The model under review builds one solid part; all positions refer to its coordinate system, in mm. Face numbers are marked on the shaded views. A direction names the side the tool comes from. Round coordinates to 2 decimals unless told otherwise and drop trailing zeros. Order: outer loops, then holes, each group sorted by start corner. A loop starts at its lowest first (then second) coordinate and runs counter-clockwise, first axis right, second up.
1) Clearance check with flat-ended pins moving along their axes: P1, Ø1.5, axis at x = 8.5, z = -4.5, coming from the -Y side; P2, Ø4.5, axis at x = -2.5, y = 0, coming from the -Z side; P3, Ø3, axis at x = -5, z = 0, coming from the -Y side; P4, Ø4, axis at x = 19.5, y = 6, coming from the +Z side. State where each tip first meets the part, or that it passes through.
2) Consider section C-C (x = 25.5). Give the boundary of the cut face in (y, z), then the cut area to 3 significant figures.
3) Consider section D-D (y = 5.75). Give the boundary of the cut face in (x, z).
4) Machinability: for the marked faces 1, 2 and 3, which of the approach directions +Z, -Z, +X, -X, +Y, -Y give a long, thin tool a straight path to every point of the face, cutting with its end or side? Answer none if there is none.
5) To check wall thickness, follow L1, parallel to Z at x = -5, y = 0.75; L2, parallel to X at y = -2, z = 5.25; L3, parallel to Z at x = 17.5, y = -0.5. State the ranges of each line that lie inside material, in increasing order.
6) Mouldability with a two-part tool opening along X and no side actions: class the marked faces 4, 5 and 6 as pulls with the +X half, pulls with the -X half, needs draft (parallel to the pull), parting line crosses it, or undercut.
7) Consider section A-A (z = 0). Give the boundary of the cut face in (x, y).
8) Consider section B-B (y = 0). Give the boundary of the cut face in (x, z), then the cut area to 3 significant figures.
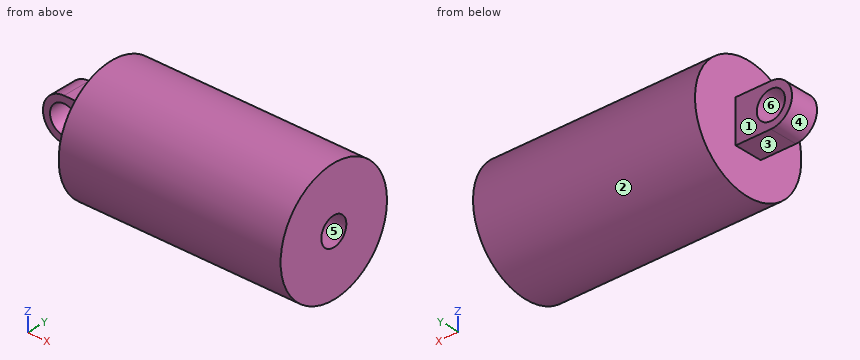
Autodesk Inventor part; units mm, degrees
ref_plane "YZ Plane" through (0, 0, 0) normal (1, 0, 0) x (0, 1, 0)
ref_plane "XZ Plane" through (0, 0, 0) normal (0, 1, 0) x (-1, 0, 0)
ref_plane "XY Plane" through (0, 0, 0) normal (0, 0, 1) x (1, 0, 0)
sketch "スケッチ1" plane through (0, 0, 0) normal (1, 0, 0) x (0, 1, 0)
  circle A0 centre (0, 0) radius 8.5
  dimension "d0" = 17
extrude "押し出し1" add sketch "スケッチ1" along normal blind 31.5
sketch "スケッチ2" plane through (0, 0, 0) normal (0, 1, 0) x (-1, 0, 0)
  circle A0 centre (5, 0) radius 2
  circle A1 centre (5, 0) radius 3
  line L0 (0, 0) -> (0, 5.5308)
  line L1 (0, 5.5308) -> (0, -7.9673)
  line L2 (5, 3) -> (0, 3)
  line L3 (5, -3) -> (0, -3)
  dimension "d3" = 4
  dimension "d4" = 5
  dimension "d5" = 6
extrude "押し出し2" add sketch "スケッチ2" along normal mid plane 4
sketch "スケッチ3" plane through (31.5, 0, 0) normal (1, 0, 0) x (0, 0, -1)
  circle A0 centre (0, 0) radius 2
  dimension "d8" = 4
extrude "押し出し3" cut sketch "スケッチ3" against normal blind 15
properties part number "black-suspension-under" material "ABS プラスチック"
Answer below:
1. P1: stops at y = -7.63
1. P2: stops at z = -3
1. P3: passes through
1. P4: stops at z = 7.5
2. outline: circle Ø17 at (0, 0); hole circle Ø4 at (0, 0)
2. area: 214 mm2
3. outline: (0, -6.26) - (31.5, -6.26) - (31.5, 6.26) - (0, 6.26) - close
4. face 1: +Z, -Z, -X, +Y
4. face 2: +X, -X
4. face 3: -Z, -X, +Y, -Y
5. L1: z = -3 to -2, 2 to 3
5. L2: x = 0 to 31.5
5. L3: z = -8.49 to -1.94, 1.94 to 8.49
6. face 4: pulls with the -X half
6. face 5: needs draft
6. face 6: undercut
7. outline: (-8, -2) - (-7, -2) - (-7, 2) - (-8, 2) - close; (-3, -2) - (0, -2) - (0, -8.5) - (31.5, -8.5) - (31.5, -2) - (16.5, -2) - (16.5, 2) - (31.5, 2) - (31.5, 8.5) - (0, 8.5) - (0, 2) - (-3, 2) - close
8. outline: (-5, -3) - (0, -3) - (0, -8.5) - (31.5, -8.5) - (31.5, -2) - (16.5, -2) - (16.5, 2) - (31.5, 2) - (31.5, 8.5) - (0, 8.5) - (0, 3) - (-5, 3) arc R3 ccw to start; hole circle Ø4 at (-5, 0)
8. area: 507 mm2
